```python
from build123d import *

# Parameters (mm, degrees)
SKETCH1_W                      = 192.4
SKETCH1_H                      = 192
BOSS_EXTRUDE1_DEPTH            = 6.35
CUT_EXTRUDE1_REACH             = 138.054
SKETCH2_W                      = 41
SKETCH2_H                      = 41
CBORE_FOR_M4_SHCS1_D           = 4.5
CBORE_FOR_M4_SHCS1_CBORE_D     = 8
CBORE_FOR_M4_SHCS1_CBORE_DEPTH = 4
SKETCH5_R                      = 2.5
CUT_EXTRUDE2_DEPTH             = 6
CUT_EXTRUDE3_REACH             = 138.038
SKETCH6_R                      = 2.25
CUT_EXTRUDE4_REACH             = 138.054
SKETCH7_R                      = 1.75
BOSS_EXTRUDE2_START            = 6
SKETCH11_R                     = 4
SKETCH11_R_2                   = 1.75
BOSS_EXTRUDE2_DEPTH            = 6
SKETCH8_R                      = 2
CUT_EXTRUDE5_DEPTH             = 5
EXTRUDE_THIN1_DEPTH            = 3
CHAMFER1_SIZE                  = 3
CHAMFER2_SIZE                  = 1


with BuildPart() as part:
    # Sketch1 → Boss-Extrude1 (new body)
    with BuildSketch(Plane(origin=(0, 0, 0), x_dir=(1, 0, 0), z_dir=(0, 1, 0))):
        Rectangle(SKETCH1_W, SKETCH1_H)
    extrude(amount=BOSS_EXTRUDE1_DEPTH)

    # Sketch2 → Cut-Extrude1 (cut, up to next)
    with BuildSketch(Plane(origin=(0, 6.35, 0), x_dir=(1, 0, 0), z_dir=(0, 1, 0)), mode=Mode.PRIVATE) as cut_extrude1_sk1:
        with Locations((-75.7, 34.5)):
            Rectangle(SKETCH2_W, SKETCH2_H)
    cut_extrude1_tool1 = extrude(cut_extrude1_sk1.sketch, amount=-CUT_EXTRUDE1_REACH, mode=Mode.PRIVATE) & part.part
    # Sketch2 → Cut-Extrude1 (cut, up to next)
    with BuildSketch(Plane(origin=(0, 6.35, 0), x_dir=(1, 0, 0), z_dir=(0, 1, 0)), mode=Mode.PRIVATE) as cut_extrude1_sk2:
        with Locations((-75.7, 75.5)):
            Rectangle(SKETCH2_W, SKETCH2_H)
    cut_extrude1_tool2 = extrude(cut_extrude1_sk2.sketch, amount=-CUT_EXTRUDE1_REACH, mode=Mode.PRIVATE) & part.part
    # Sketch2 → Cut-Extrude1 (cut, up to next)
    with BuildSketch(Plane(origin=(0, 6.35, 0), x_dir=(1, 0, 0), z_dir=(0, 1, 0)), mode=Mode.PRIVATE) as cut_extrude1_sk3:
        with Locations((-34.7, 75.5)):
            Rectangle(SKETCH2_W, SKETCH2_H)
    cut_extrude1_tool3 = extrude(cut_extrude1_sk3.sketch, amount=-CUT_EXTRUDE1_REACH, mode=Mode.PRIVATE) & part.part
    add(cut_extrude1_tool1.solids().sort_by_distance((-75.7, 6.35, -34.5))[0], mode=Mode.SUBTRACT)
    add(cut_extrude1_tool2.solids().sort_by_distance((-75.7, 6.35, -75.5))[0], mode=Mode.SUBTRACT)
    add(cut_extrude1_tool3.solids().sort_by_distance((-34.7, 6.35, -75.5))[0], mode=Mode.SUBTRACT)

    # CBORE for M4 SHCS1 (through all)
    with Locations(Plane(origin=(0, 6.35, 0), x_dir=(1, 0, 0), z_dir=(0, 1, 0))):
        with Locations((76.2, 76), (-76.2, -4), (-76.2, -76), (3.8, 76)):
            CounterBoreHole(CBORE_FOR_M4_SHCS1_D / 2, CBORE_FOR_M4_SHCS1_CBORE_D / 2, CBORE_FOR_M4_SHCS1_CBORE_DEPTH)

    # Sketch5 → Cut-Extrude2 (cut)
    with BuildSketch(Plane(origin=(0, 6.35, 0), x_dir=(1, 0, 0), z_dir=(0, 1, 0))):
        with Locations(Location((-18.7, -8.525, 0), (0, 0, 270))):
            Circle(SKETCH5_R)
        with Locations(Location((-18.7, -73.475, 0), (0, 0, 270))):
            Circle(SKETCH5_R)
    extrude(amount=-CUT_EXTRUDE2_DEPTH, mode=Mode.SUBTRACT)

    # Sketch6 → Cut-Extrude3 (cut, up to next)
    with BuildSketch(Plane(origin=(0, 0.35, 0), x_dir=(1, 0, 0), z_dir=(0, 1, 0)), mode=Mode.PRIVATE) as cut_extrude3_sk1:
        with Locations(Location((-18.7, -8.525, 0), (0, 0, 270))):
            Circle(SKETCH6_R)
    cut_extrude3_tool1 = extrude(cut_extrude3_sk1.sketch, amount=-CUT_EXTRUDE3_REACH, mode=Mode.PRIVATE) & part.part
    # Sketch6 → Cut-Extrude3 (cut, up to next)
    with BuildSketch(Plane(origin=(0, 0.35, 0), x_dir=(1, 0, 0), z_dir=(0, 1, 0)), mode=Mode.PRIVATE) as cut_extrude3_sk2:
        with Locations(Location((-18.7, -73.475, 0), (0, 0, 270))):
            Circle(SKETCH6_R)
    cut_extrude3_tool2 = extrude(cut_extrude3_sk2.sketch, amount=-CUT_EXTRUDE3_REACH, mode=Mode.PRIVATE) & part.part
    add(cut_extrude3_tool1.solids().sort_by_distance((-18.7, 0.35, 8.525))[0], mode=Mode.SUBTRACT)
    add(cut_extrude3_tool2.solids().sort_by_distance((-18.7, 0.35, 73.475))[0], mode=Mode.SUBTRACT)

    # Sketch7 → Cut-Extrude4 (cut, up to next)
    with BuildSketch(Plane(origin=(0, 6.35, 0), x_dir=(1, 0, 0), z_dir=(0, 1, 0)), mode=Mode.PRIVATE) as cut_extrude4_sk1:
        with Locations(Location((21.2, 61, 0), (0, 0, 270))):
            Circle(SKETCH7_R)
    cut_extrude4_tool1 = extrude(cut_extrude4_sk1.sketch, amount=-CUT_EXTRUDE4_REACH, mode=Mode.PRIVATE) & part.part
    # Sketch7 → Cut-Extrude4 (cut, up to next)
    with BuildSketch(Plane(origin=(0, 6.35, 0), x_dir=(1, 0, 0), z_dir=(0, 1, 0)), mode=Mode.PRIVATE) as cut_extrude4_sk2:
        with Locations(Location((21.2, 17.5, 0), (0, 0, 270))):
            Circle(SKETCH7_R)
    cut_extrude4_tool2 = extrude(cut_extrude4_sk2.sketch, amount=-CUT_EXTRUDE4_REACH, mode=Mode.PRIVATE) & part.part
    add(cut_extrude4_tool1.solids().sort_by_distance((21.2, 6.35, -61))[0], mode=Mode.SUBTRACT)
    add(cut_extrude4_tool2.solids().sort_by_distance((21.2, 6.35, -17.5))[0], mode=Mode.SUBTRACT)

    # Sketch11 → Boss-Extrude2 (add)
    # profile 1 of 2: a face of its own
    with BuildSketch(Plane(origin=(0, 6.35, 0), x_dir=(1, 0, 0), z_dir=(0, 1, 0)).offset(BOSS_EXTRUDE2_START)):
        with Locations(Location((21.2, 61, 0), (0, 0, 270))):
            Circle(SKETCH11_R)
        with Locations(Location((21.2, 61, 0), (0, 0, 270))):
            Circle(SKETCH11_R_2, mode=Mode.SUBTRACT)
    # profile 2 of 2: a face of its own
    with BuildSketch(Plane(origin=(0, 6.35, 0), x_dir=(1, 0, 0), z_dir=(0, 1, 0)).offset(BOSS_EXTRUDE2_START)):
        with Locations(Location((21.2, 17.5, 0), (0, 0, 270))):
            Circle(SKETCH11_R)
        with Locations(Location((21.2, 17.5, 0), (0, 0, 270))):
            Circle(SKETCH11_R_2, mode=Mode.SUBTRACT)
    extrude(amount=-BOSS_EXTRUDE2_DEPTH)

    # Sketch8 → Cut-Extrude5 (cut)
    with BuildSketch(Plane(origin=(0, 12.35, 0), x_dir=(1, 0, 0), z_dir=(0, 1, 0))):
        with Locations(Location((21.2, 61, 0), (0, 0, 270))):
            Circle(SKETCH8_R)
        with Locations(Location((21.2, 17.5, 0), (0, 0, 270))):
            Circle(SKETCH8_R)
    extrude(amount=-CUT_EXTRUDE5_DEPTH, mode=Mode.SUBTRACT)

    # Sketch9 → Extrude-Thin1 (add)
    with BuildSketch(Plane(origin=(0, 6.35, 0), x_dir=(1, 0, 0), z_dir=(0, 1, 0))):
        Polygon((-96.2, -89.5), (89.7, -89.5), (89.7, 0), (86.7, 0), (86.7, -86.5), (-96.2, -86.5), align=None)
    extrude(amount=EXTRUDE_THIN1_DEPTH)

    # Chamfer1
    chamfer1_edges = [part.edges().sort_by_distance(p)[0] for p in [
        (-4.75, 6.35, 86.5),
        (86.7, 6.35, 43.25),
        (-3.25, 6.35, 89.5),
        (89.7, 6.35, 44.75),
    ]]
    chamfer(chamfer1_edges, length=CHAMFER1_SIZE - 0.0001)  # a hair under: the kernel refuses the full size

    # Chamfer2
    chamfer2_edges = [part.edges().sort_by_distance(p)[0] for p in [
        (0, 0, 96),
        (96.2, 0, 0),
    ]]
    chamfer(chamfer2_edges, length=CHAMFER2_SIZE)


solid = part.part
```
For this review, take the finished solid that the model builds, in its own axes (mm). A direction names the side the tool comes from. Coordinates: 2 decimals unless noted, no trailing zeros.
(1) Add section A-A on x = -18.7. Count the separate pieces of the cut face and the enclosed holes in it, then the cut area to 3 significant figures.
(2) Tool access review of faces 3 (the face through (75.162, 1.159, -74.004)), 4 (the face through (-80.196, 4.378, 3.824)), 5 (the face through (-55.2, 3, -34)): name each direction out of +Z, -Z, +X, -X, +Y, -Y from which nothing blocks a thin tool from reaching the whole face with its end or side.
(3) For pin 1 Ø6 at (x, y) = (-45, 3) entering from -Z; pin 2 Ø2 at (x, z) = (-59.5, 10) entering from +Y; pin 3 Ø7 at (x, z) = (-76.2, 4) entering from +Y; pin 4 Ø3 at (x, z) = (21.2, -17.5) entering from +Y, all flat-tipped, find the tip position at first contact; note any pin that passes through.
(4) The part is to be moulded in two halves that separate along Z. For faces 1 (the face through (78.046, 4.378, -72.451)), 2 (the face through (96.2, 4, 1)), say which applies: +Z half, -Z half, draft (parallel to the pull), parting line (faces both ways), or undercut.
(5) Wall thickness on probe 1 along Z at (x, y) = (-76.2, 1.3); probe 2 along X at (y, z) = (10.5, -17.5); probe 3 along Y at (x, z) = (-6.5, -53.5): over which ranges is each line inside the solid? List them lowest first.
Answer sheet:
1. separate pieces: 3
1. enclosed holes: 0
1. area: 913 mm2
2. face 3: +Y, -Y
2. face 4: +Y
2. face 5: -Z, -X, +Y, -Y
3. pin 1: stops at z = -55
3. pin 2: stops at y = 6.35
3. pin 3: stops at y = 2.35
3. pin 4: passes through
4. face 1: undercut
4. face 2: draft
5. probe 1: z = -14 to 1.75, 6.25 to 73.75, 78.25 to 96
5. probe 2: x = 17.2 to 19.2, 23.2 to 25.2
5. probe 3: y = 0 to 6.35
